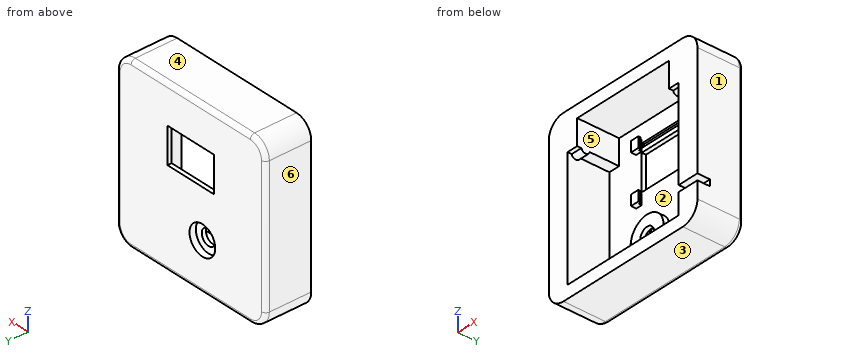
Autodesk Inventor part; units mm, degrees
ref_plane "YZ Plane" through (0, 0, 0) normal (1, 0, 0) x (0, 1, 0)
ref_plane "XZ Plane" through (0, 0, 0) normal (0, 1, 0) x (-1, 0, 0)
ref_plane "XY Plane" through (0, 0, 0) normal (0, 0, 1) x (1, 0, 0)
sketch "Skizze1" plane through (0, 0, 0) normal (0, 1, 0) x (-1, 0, 0)
  line L0 (30.3, 19.3) -> (-30.3, 19.3)
  line L1 (-30.3, 19.3) -> (-30.3, -34.9)
  line L2 (-30.3, -34.9) -> (30.3, -34.9)
  line L3 (30.3, -34.9) -> (30.3, 19.3)
  line L4 (40.5, -43.7) -> (-40.5, -43.7)
  line L5 (-40.5, -43.7) -> (-40.5, 37.3)
  line L6 (-40.5, 37.3) -> (40.5, 37.3)
  line L7 (40.5, 37.3) -> (40.5, -43.7)
  point P0 (0, 0)
  dimension "d0" = 30.3
  dimension "d1" = 60.6
  dimension "d2" = 54.2
  dimension "d3" = 19.3
  dimension "d4" = 81
  dimension "d5" = 81
  dimension "d6" = 40.5
  dimension "d7" = 18
extrude "Extrusion1" add sketch "Skizze1" along normal blind 20
sketch "Skizze2" plane through (0, 0, 0) normal (0, -1, 0) x (1, 0, 0)
  line L0 (-40.5, 37.3) -> (40.5, 37.3)
  line L1 (40.5, 37.3) -> (40.5, -43.7)
  line L2 (40.5, -43.7) -> (-40.5, -43.7)
  line L3 (-40.5, -43.7) -> (-40.5, 37.3)
  point P0 (0, 0)
sketch "Skizze3" plane through (0, 20, 0) normal (0, 1, 0) x (1, 0, 0)
  line L0 (30.3, -19.3) -> (-30.3, -19.3)
  line L1 (25, -19.3) -> (-25, -19.3)
  line L2 (-25, -19.3) -> (-25, -31.3)
  line L3 (-25, -31.3) -> (25, -31.3)
  line L4 (25, -31.3) -> (25, -19.3)
  point P0 (0, 0)
  point P1 (-25, -19.3)
  dimension "d12" = 12
  dimension "d13" = 50
  dimension "d14" = 25
extrude "Extrusion3" cut sketch "Skizze3" against normal blind 20
sketch "Skizze4" plane through (0, 20, 0) normal (0, 1, 0) x (1, 0, 0)
  line L0 (-40.5, -37.3) -> (40.5, -37.3)
  line L1 (-40.5, 43.7) -> (-40.5, -37.3)
  line L2 (40.5, -37.3) -> (-40.5, -37.3)
  line L3 (-40.5, -37.3) -> (-40.5, 43.7)
  line L4 (-40.5, 43.7) -> (40.5, 43.7)
  line L5 (40.5, 43.7) -> (40.5, -37.3)
  point P0 (0, 0)
extrude "Extrusion4" add sketch "Skizze4" along normal blind 2
sketch "Skizze5" plane through (0, 20, 0) normal (0, -1, 0) x (1, 0, 0)
  line L0 (-12.7, 19) -> (12.7, 19)
  line L1 (12.7, 19) -> (12.7, 2)
  line L2 (12.7, 2) -> (-12.7, 2)
  line L3 (-12.7, 2) -> (-12.7, 19)
  point P0 (0, 0)
  dimension "d19" = 25.4
  dimension "d20" = 17
  dimension "d21" = 12.7
  dimension "d22" = 2
extrude "Extrusion5" cut sketch "Skizze5" against normal blind 20
sketch "Skizze6" plane through (0, 20, 0) normal (0, -1, 0) x (1, 0, 0)
  line L0 (-12.5757, 21) -> (12.5757, 21)
  line L1 (12.5757, 21) -> (12.5757, 23)
  line L2 (12.5757, 23) -> (-12.5757, 23)
  line L3 (-12.5757, 23) -> (-12.5757, 21)
  line L4 (-12.7, 19) -> (12.7, 19)
  point P0 (0, 0)
  dimension "d25" = 2
  dimension "d26" = 2
extrude "Extrusion6" cut sketch "Skizze6" against normal blind 1
sketch "Skizze7" plane through (0, 20, 0) normal (0, -1, 0) x (1, 0, 0)
  line L0 (-15.7, -3.5) -> (-11.7, -3.5)
  line L1 (-11.7, -3.5) -> (-11.7, 1.5)
  line L2 (-11.7, 1.5) -> (-15.7, 1.5)
  line L3 (-15.7, 1.5) -> (-15.7, -3.5)
  line L4 (-15.7, 19.5) -> (-11.7, 19.5)
  line L5 (-11.7, 19.5) -> (-11.7, 24.5)
  line L6 (-11.7, 24.5) -> (-15.7, 24.5)
  line L7 (-15.7, 24.5) -> (-15.7, 19.5)
  line L8 (12.7, 2) -> (-12.7, 2)
  line L9 (-12.7, 19) -> (12.7, 19)
  line L10 (-12.7, 2) -> (-12.7, 19)
  point P0 (0, 0)
  point P1 (-11.7, 22)
  dimension "d29" = 4
  dimension "d30" = 0.5
  dimension "d31" = 5
  dimension "d32" = 5
  dimension "d33" = 0.5
  dimension "d34" = 1
extrude "Extrusion7" add sketch "Skizze7" along normal blind 2.5
sketch "Skizze8" plane through (-11.7, 20, -3.5) normal (0, 0, -1) x (-1, 0, 0)
  line L0 (0, 0) -> (0, -2.5)
  line L1 (0, 0) -> (1, 0)
  line L2 (1, 0) -> (1, -1.4)
  line L3 (1, -1.4) -> (0, -1.4)
  line L4 (0, -1.4) -> (0, 0)
  point P0 (-11.7, -20)
  point P1 (0, -1.4)
  dimension "d37" = 1
  dimension "d38" = 1.4
extrude "Extrusion8" cut sketch "Skizze8" against normal blind 29.5
fillet "Rundung1" radius 8 4 edges at (40.5, 11, 37.3) (40.5, 11, -43.7) (-40.5, 11, 37.3) (-40.5, 11, -43.7)
fillet "Rundung2" radius 2 8 edges at (38.1569, 22, -41.3569) (0, 22, -43.7) (-38.1569, 22, -41.3569) (-40.5, 22, -3.2) (-38.1569, 22, 34.9569) (0, 22, 37.3) (38.1569, 22, 34.9569) (40.5, 22, -3.2)
sketch "Skizze9" plane through (-30.3, 0, 19.3) normal (1, 0, 0) x (0, 0, -1)
  line L0 (54, 11) -> (57, 0)
  line L1 (63, 0) -> (55, 0)
  line L2 (57, 0) -> (54, 0)
  line L3 (54, 0) -> (54, 11)
  line L4 (53.8, 6) -> (53.8, 11)
  line L5 (53.8, 6) -> (53.8, 2)
  line L6 (49.8, 6) -> (53.8, 6)
  line L7 (49.8, 2) -> (49.8, 6)
  line L8 (49.8, 2) -> (53.8, 2)
  line L9 (49.8, 6) -> (53.8, 6)
  line L10 (53.8, 6) -> (53.8, 11)
  line L11 (49.8, 11) -> (53.8, 11)
  line L12 (49.8, 8.9) -> (49.8, 11)
  line L13 (49.8, 8.9) -> (51.8, 8.9)
  line L14 (51.8, 8.9) -> (51.8, 7)
  line L15 (51.8, 7) -> (49.8, 7)
  line L16 (49.8, 6) -> (49.8, 7)
  point P0 (19.3, 0)
  dimension "d45" = 11
  dimension "d46" = 9
  dimension "d47" = 3
extrude "Extrusion9" cut sketch "Skizze9" along normal up to surface (60.6 mm away) contours L0 L1 L2 L3
sketch "Skizze10" plane through (-25, 0, 31.3) normal (1, 0, 0) x (0, 0, -1)
  line L0 (16.3, 6) -> (12.3, 6)
  line L1 (12.3, 2) -> (31.3, 2)
  line L2 (12, 0) -> (12, 20)
  arc A0 (12, 2) -> (12, 6) centre (11.4824, 4) ccw
  line L3 (12, 2) -> (12, 6)
  point P0 (31.3, 0)
extrude "Extrusion10" add sketch "Skizze10" against normal blind 10
sketch "Skizze11" plane through (25, 0, 19.3) normal (-1, 0, 0) x (0, 0, 1)
  line L0 (12, 20) -> (0, 20)
  line L1 (12, 20) -> (12, 0)
  line L2 (0, 0) -> (12, 0)
  line L3 (0, 2) -> (0, 0)
  arc A0 (0, 6) -> (0, 2) centre (0.5176, 4) ccw
  line L4 (0, 20) -> (0, 6)
  line L5 (0, 6) -> (0, 2)
  line L6 (0, 0) -> (0, 20)
  arc A1 (0, 2) -> (0, 2) centre (0.512, 3.9787) ccw
  point P0 (-19.3, 0)
extrude "Extrusion11" add sketch "Skizze11" against normal blind 10 contours A0 L5 A1 | A1 L5 picked at (-0.1516, 3.3785)
sketch "Skizze12" plane through (0, 20, 0) normal (0, -1, 0) x (1, 0, 0)
  circle A0 centre (-6.3, -20.9) radius 3.75
  line L0 (-30.3, -34.9) -> (30.3, -34.9)
  line L1 (-30.3, 19.3) -> (-30.3, -37.7)
  point P0 (0, 0)
  dimension "d52" = 14
  dimension "d53" = 24
  dimension "d54" = 7.5
extrude "Extrusion12" cut sketch "Skizze12" against normal blind 10
sketch "Skizze13" plane through (0, 20, 0) normal (0, -1, 0) x (1, 0, 0)
  circle A0 centre (-6.3, -20.9) radius 4.75
  circle A1 centre (-6.3, -20.9) radius 9
  point P0 (0, 0)
  dimension "d57" = 18
  dimension "d70" = 9.5
extrude "Extrusion13" add sketch "Skizze13" along normal blind 3 contours A0 | A1
sketch "Skizze14" plane through (-6.3, 20, -20.9) normal (0, 1, 0) x (1, 0, 0)
  circle A0 centre (0, 0) radius 3.75
  point P0 (6.3, -20.9)
extrude "Extrusion14" cut sketch "Skizze14" against normal through all
sketch "Skizze15" plane through (0, 22, 0) normal (0, 1, 0) x (1, 0, 0)
  circle A0 centre (-6.3, 20.9) radius 3.75
  circle A1 centre (-6.3, 20.9) radius 7
  point P0 (0, 0)
  dimension "d62" = 14
extrude "Extrusion15" cut sketch "Skizze15" against normal blind 3
sketch "Skizze16" plane through (40.5, 0, 29.3) normal (1, 0, 0) x (0, 0, -1)
  line L0 (67, 0) -> (10, 0)
  line L1 (54, 0) -> (57, 0)
  line L2 (57, 0) -> (57, 6)
  line L3 (57, 6) -> (54, 6)
  line L4 (54, 6) -> (54, 0)
  line L5 (73, 0) -> (73, 20)
  point P0 (29.3, 0)
  dimension "d65" = 6
  dimension "d66" = 3
  dimension "d67" = 16
extrude "Extrusion16" cut sketch "Skizze16" against normal blind 27.75
properties part number "Deckel"
The model under review builds one solid part; all positions refer to its coordinate system, in mm. Face numbers are marked on the shaded views. A direction names the side the tool comes from. Round coordinates to 2 decimals unless told otherwise and drop trailing zeros. Write each loop counter-clockwise with the first axis right and the second up, starting at its lowest first coordinate (ties: lowest second). Pieces come first, ordered by that corner, then holes. Notation, with made-up numbers: M 35,-35.75 L 82,-35.75 A28 ccw 82,-16.75 Z; hole C 81,3 d2. An arc over 180 degrees is marked long. Use a Markdown table: item, result. Add a question column.
Q1. To check wall thickness, follow line 1 (Z direction, x = -6.3, y = 20.3); line 2 (X direction, y = 18, z = 22.5); line 3 (X direction, y = 5.25, z = 11). State the ranges of each line that lie inside material, in increasing order.
Q2. We need section A-A, the plane x = -6.3. Count the separate pieces of the cut face and the enclosed holes in it, plus the area to 3 significant figures.
Q3. We need section D-D, the plane x = 18. State the section outline as (y, z) points.
Q4. We need section B-B, the plane z = 4.5. State the section outline as (x, y) points.
Q5. The part is to be moulded in two halves that separate along Z. For the marked faces 1, 2, 3 and 4, say which applies: pulls with the +Z half, pulls with the -Z half, needs draft (parallel to the pull), parting line crosses it, or undercut.
Q6. Machinability: for the marked faces 5 and 6, which of the approach directions +Z, -Z, +X, -X, +Y, -Y give a long, thin tool a straight path to every point of the face, cutting with its end or side? Answer none if there is none.
Q7. We need section C-C, the plane z = -7.5. State the section outline as (x, y) points.
Q8. Insertion check: pin 1 (10 mm diameter, centred on x = 7, z = -21.5, fed in from -Y); pin 2 (8.5 mm diameter, centred on x = -6.3, z = -20.9, fed in from +Y); pin 3 (2 mm diameter, centred on x = -14.5, z = -1.5, fed in from -Y). Each pin has a flat end and moves straight along its axis. Give the tip position at first contact, or say it passes through.
Findings below:
| question | item | result |
|---|---|---|
| 1 | line 1 | z = -43.68 to -27.9, -13.9 to 2, 19 to 21, 23 to 37.28 |
| 1 | line 2 | x = -40.5 to -25, -15.7 to -11.7, 25 to 40.5 |
| 1 | line 3 | x = -40.5 to -30.3, 30.3 to 40.5 |
| 2 | separate pieces | 3 |
| 2 | enclosed holes | 0 |
| 2 | area | 403 mm² |
| 3 | outline | M 0,-43.7 L 20,-43.7 A2 ccw 22,-41.7 L 22,35.3 A2 ccw 20,37.3 L 0,37.3 L 0,31.3 L 20,31.3 L 20,-34.9 L 10.27,-34.9 L 0,-37.7 Z |
| 4 | outline | M -40.5,0 L -30.3,0 L -30.3,20 L -12.7,20 L -12.7,22 L -38.5,22 A2 ccw -40.5,20 Z; M 12.7,20 L 30.3,20 L 30.3,0 L 40.5,0 L 40.5,20 A2 ccw 38.5,22 L 12.7,22 Z |
| 5 | face 1 | needs draft |
| 5 | face 2 | undercut |
| 5 | face 3 | pulls with the -Z half |
| 5 | face 4 | pulls with the +Z half |
| 6 | face 5 | -Y |
| 6 | face 6 | +Z, -Z, -X, +Y, -Y |
| 7 | outline | M -40.5,0 L -30.3,0 L -30.3,20 L 30.3,20 L 30.3,0 L 40.5,0 L 40.5,20 A2 ccw 38.5,22 L -38.5,22 A2 ccw -40.5,20 Z |
| 8 | pin 1 | stops at y = 17 |
| 8 | pin 2 | stops at y = 19 |
| 8 | pin 3 | stops at y = 17.5 |
